The listing builds one solid part. Answer for the finished solid, in the listing's coordinates (mm). Coordinates: 2 decimals unless noted, no trailing zeros. Write each loop counter-clockwise with the first axis right and the second up, starting at its lowest first coordinate (ties: lowest second). Pieces come first, ordered by that corner, then holes.
from build123d import *

# Parameters (mm, degrees)
SKETCH1_W                  = 3
SKETCH1_H                  = 10.1
SKETCH2_R                  = 3.5
BOSS_EXTRUDE1_DEPTH        = 1
DOME1_FACE_RADIUS          = 3.5
DOME1_HEIGHT               = 1
MIRROR1_COPY_1_FACE_RADIUS = 3.5
MIRROR1_COPY_1_HEIGHT      = 1


with BuildPart() as part:
    # Sketch1 → Revolve1 (revolve)
    with BuildSketch(Plane.XY, mode=Mode.PRIVATE) as revolve1_sk:
        with Locations((-1.5, 5.05)):
            Rectangle(SKETCH1_W, SKETCH1_H)
    revolve1 = revolve(revolve1_sk.sketch.rotate(Axis((0, 5.950819672, 0), (0, -1, 0)), 270), axis=Axis((0, 5.950819672, 0), (0, -1, 0)))

    # Sketch2 → Boss-Extrude1 (add)
    with BuildSketch(Plane(origin=(0, 10.1, 0), x_dir=(1, 0, 0), z_dir=(0, 1, 0))):
        with Locations(Location((0, 0, 0), (0, 0, 270))):
            Circle(SKETCH2_R)
    boss_extrude1 = extrude(amount=BOSS_EXTRUDE1_DEPTH)

    # Dome1: a dome of height H over a round flat face of radius A is a cap of a sphere of radius (A * A + H * H) / (2 * H)
    dome1_r = (DOME1_FACE_RADIUS * DOME1_FACE_RADIUS + DOME1_HEIGHT * DOME1_HEIGHT) / (2 * DOME1_HEIGHT)
    dome1_base = Plane((0, 11.1, 0), z_dir=(0, 1, 0))
    with Locations(dome1_base.offset(DOME1_HEIGHT - dome1_r)):
        dome1_ball = Sphere(dome1_r, mode=Mode.PRIVATE)
    add(split(dome1_ball, bisect_by=dome1_base, keep=Keep.TOP, mode=Mode.PRIVATE))

    # Mirror1: Revolve1, Boss-Extrude1 across plane
    add(revolve1.mirror(Plane.ZX))
    add(boss_extrude1.mirror(Plane.ZX))

    # Mirror1 copy 1: a dome of height H over a round flat face of radius A is a cap of a sphere of radius (A * A + H * H) / (2 * H)
    mirror1_copy_1_r = (MIRROR1_COPY_1_FACE_RADIUS * MIRROR1_COPY_1_FACE_RADIUS + MIRROR1_COPY_1_HEIGHT * MIRROR1_COPY_1_HEIGHT) / (2 * MIRROR1_COPY_1_HEIGHT)
    mirror1_copy_1_base = Plane((0, -11.1, 0), z_dir=(0, -1, 0))
    with Locations(mirror1_copy_1_base.offset(MIRROR1_COPY_1_HEIGHT - mirror1_copy_1_r)):
        mirror1_copy_1_ball = Sphere(mirror1_copy_1_r, mode=Mode.PRIVATE)
    add(split(mirror1_copy_1_ball, bisect_by=mirror1_copy_1_base, keep=Keep.TOP, mode=Mode.PRIVATE))


solid = part.part
1. Flat-ended cylindrical pins translate along their axes: P1, Ø1, axis at x = 1.5, z = 2.5, coming from the +Y side; P2, Ø3, axis at y = -4.5, z = -1.5, coming from the -X side; P3, Ø1, axis at x = 1, z = 1, coming from the -Y side. Find the tip coordinate at first contact, or state that the pin passes through.
Results found:
P1: stops at y = 11.64
P2: stops at x = -3
P3: stops at y = -12.04
2. Section A-A on z = 0 is taken. Give the vertices of the cut face in (x, y) (3 decimals).
Results found:
outline: (-3.5, -11.1) arc R6.625 ccw to (3.5, -11.1) - (3.5, -10.1) - (3, -10.1) - (3, 10.1) - (3.5, 10.1) - (3.5, 11.1) arc R6.625 ccw to (-3.5, 11.1) - (-3.5, 10.1) - (-3, 10.1) - (-3, -10.1) - (-3.5, -10.1) - close
3. Section D-D on y = 7 is taken. Give the vertices of the cut face in (x, z).
Results found:
outline: circle Ø6 at (0, 0)
4. Find the intervals of material crossed by L1, parallel to Y at x = 3, z = 0.5; L2, parallel to X at y = -1.75, z = -0.75; L3, parallel to Z at x = 2, y = -5.75, in increasing order.
Results found:
L1: y = -11.36 to -10.1, 10.1 to 11.36
L2: x = -2.9 to 2.9
L3: z = -2.24 to 2.24
5. Section C-C on y = 10.75 is taken. Give the vertices of the cut face in (x, z), then the cut area to 3 significant figures.
Results found:
outline: circle Ø7 at (0, 0)
area: 38.5 mm2
6. Section B-B on x = 0 is taken. Give the vertices of the cut face in (y, z) (3 decimals).
Results found:
outline: (-11.1, -3.5) - (-10.1, -3.5) - (-10.1, -3) - (10.1, -3) - (10.1, -3.5) - (11.1, -3.5) arc R6.625 ccw to (11.1, 3.5) - (10.1, 3.5) - (10.1, 3) - (-10.1, 3) - (-10.1, 3.5) - (-11.1, 3.5) arc R6.625 ccw to start
7. For a pull along Y with two mould halves and no side action, classify faces 1 (the flat face through (1, -10.1, 3)), 2 (the flat face through (1, 10.1, 3)), 3 (the cylindrical face through (-3.417, 10.593, -0.759)) as pulls with the +Y half, pulls with the -Y half, needs draft (parallel to the pull), parting line crosses it, or undercut.
Results found:
face 1: undercut
face 2: undercut
face 3: needs draft
